```python
from build123d import *

# Parameters (mm, degrees)
SKETCH009_W          = 140
SKETCH009_H          = 120
PAD004_DEPTH         = 14
POCKET005_DEPTH      = 12
SKETCH011_R          = 1.75
POCKET006_DEPTH      = 0.001
POCKET006_DEPTH_BACK = 14.001
SKETCH012_R          = 4
POCKET007_DEPTH      = 12.001
SKETCH013_R          = 1.75
POCKET008_DEPTH      = 14.001


with BuildPart() as part:
    # Sketch009 → Pad004 (new body)
    with BuildSketch(Plane.XY):
        with Locations((-11.165, 15.85)):
            Rectangle(SKETCH009_W, SKETCH009_H)
    extrude(amount=PAD004_DEPTH)

    # Sketch010 → Pocket005 (cut)
    with BuildSketch(Plane.XY):
        with BuildLine():
            ThreePointArc((-79.165, 60.35), (-69.619058, 64.304058), (-65.665, 73.85))
            Line((43.335, 73.85), (-65.665, 73.85))
            ThreePointArc((43.335, 73.85), (47.289058, 64.304058), (56.835, 60.35))
            Line((56.835, -42.15), (56.835, 60.35))
            Line((-65.665, -42.15), (56.835, -42.15))
            ThreePointArc((-65.665, -42.15), (-69.619058, -32.604058), (-79.165, -28.65))
            Line((-79.165, 60.35), (-79.165, -28.65))
        make_face()
    extrude(amount=POCKET005_DEPTH, mode=Mode.SUBTRACT)

    # Sketch011 → Pocket006 (cut, two sides)
    with BuildSketch(Plane.XY) as pocket006_sk:
        with Locations((-74, 68)):
            Circle(SKETCH011_R)
        with Locations((52, 68)):
            Circle(SKETCH011_R)
        with Locations((-74, -37)):
            Circle(SKETCH011_R)
    extrude(amount=-POCKET006_DEPTH, mode=Mode.SUBTRACT)
    extrude(pocket006_sk.sketch, amount=POCKET006_DEPTH_BACK, mode=Mode.SUBTRACT)

    # Sketch012 (on DatumPlane) → Pocket007 (cut, through all)
    with BuildSketch(Plane.XY.offset(2)):
        with Locations((-74, 68)):
            Circle(SKETCH012_R)
        with Locations((52, 68)):
            Circle(SKETCH012_R)
        with Locations((-74, -37)):
            Circle(SKETCH012_R)
    extrude(amount=POCKET007_DEPTH, mode=Mode.SUBTRACT)

    # Sketch013 → Pocket008 (cut, through all)
    with BuildSketch(Plane.XY):
        with Locations((-36, 41)):
            Circle(SKETCH013_R)
        with Locations((-4, 41)):
            Circle(SKETCH013_R)
        with Locations((-36, 9)):
            Circle(SKETCH013_R)
        with Locations((-4, 9)):
            Circle(SKETCH013_R)
        with BuildLine():
            ThreePointArc((-40.582576, 39), (-32.464466, 37.464466), (-34, 45.582576))
            Line((-34, 45.582576), (-6, 45.582576))
            ThreePointArc((-6, 45.582576), (-7.535534, 37.464466), (0.582576, 39))
            Line((0.582576, 39), (0.582576, 11))
            ThreePointArc((0.582576, 11), (-7.535534, 12.535534), (-6, 4.417424))
            Line((-6, 4.417424), (-34, 4.417424))
            ThreePointArc((-34, 4.417424), (-32.464466, 12.535534), (-40.582576, 11))
            Line((-40.582576, 39), (-40.582576, 11))
        make_face()
    extrude(amount=POCKET008_DEPTH, mode=Mode.SUBTRACT)


with BuildPart() as part_1:
    # Body001 placement: moved
    add(part.part.moved(Location((0, 0, 32))))


solid = part_1.part
```
Geometry check sheet. Reference: the model listing, model coordinates, mm. A direction names the side the tool comes from. Round coordinates to 2 decimals unless told otherwise and drop trailing zeros. Write each loop counter-clockwise with the first axis right and the second up, starting at its lowest first coordinate (ties: lowest second). Pieces come first, ordered by that corner, then holes. Notation, with made-up numbers: (70.5, -4) - (120.5, -4) arc R17 ccw to (120.5, 3) - close; hole circle Ø10 at (82.25, 64). An arc over 180 degrees is marked (long way). Write each question's results on one line, items separated by ' | '.
(1) Sectioned sample at D-D, the plane x = -62. Enter the section's corners in (y, z).
Computed:
outline: (-44.15, 32) - (-42.15, 32) - (-42.15, 44) - (73.85, 44) - (73.85, 32) - (75.85, 32) - (75.85, 46) - (-44.15, 46) - close
(2) Sectioned sample at A-A, the plane x = -36. Enter the section's corners in (y, z), plus the area to 3 significant figures.
Computed:
outline: (-44.15, 32) - (-42.15, 32) - (-42.15, 44) - (7.25, 44) - (7.25, 46) - (-44.15, 46) - close; (10.75, 44) - (14, 44) - (14, 46) - (10.75, 46) - close; (36, 44) - (39.25, 44) - (39.25, 46) - (36, 46) - close; (42.75, 44) - (73.85, 44) - (73.85, 32) - (75.85, 32) - (75.85, 46) - (42.75, 46) - close | area: 230 mm^2
(3) Depth check by flat-ended pin: pin 1 Ø8 at (x, y) = (30, 12.5) entering from -Z; pin 2 Ø9 at (x, y) = (52, 68) entering from -Z; pin 3 Ø3 at (x, y) = (52, 68) entering from -Z; pin 4 Ø5.5 at (x, y) = (-74, 68) entering from +Z. Enter the tip coordinate at first touch or a pass-through.
Computed:
pin 1: stops at z = 44 | pin 2: stops at z = 32 | pin 3: passes through | pin 4: stops at z = 34
(4) Set-up check for faces 1 (the face through (51.133, 64.095, 39.916)), 2 (the face through (-72.331, -36.474, 32.986)), 3 (the face through (-10, 73.85, 38)): record each of +Z, -Z, +X, -X, +Y, -Y from which the full face is reachable in a straight line by a thin tool's end or side.
Computed:
face 1: +Z | face 2: +Z, -Z | face 3: -Z
(5) Sectioned sample at C-C, the plane y = 68. Enter the section's corners in (x, z) (3 decimals), plus the area to 3 significant figures.
Computed:
outline: (-81.165, 32) - (-75.75, 32) - (-75.75, 34) - (-78, 34) - (-78, 46) - (-81.165, 46) - close; (-72.25, 32) - (-66.998, 32) - (-66.998, 44) - (44.668, 44) - (44.668, 32) - (50.25, 32) - (50.25, 34) - (48, 34) - (48, 46) - (-70, 46) - (-70, 34) - (-72.25, 34) - close; (53.75, 32) - (58.835, 32) - (58.835, 46) - (56, 46) - (56, 34) - (53.75, 34) - close | area: 414 mm^2
(6) Thickness scan on probe 1 along Y at (x, z) = (-4, 44.65); probe 2 along X at (y, z) = (57, 38.25) (3 decimals); probe 3 along Y at (x, z) = (-23.5, 45.25). Record the ranges inside material, lowest first. Write a range as from..to.
Computed:
probe 1: y = -44.15..7.25, 10.75..14, 36..39.25, 42.75..75.85 | probe 2: x = -81.165..-79.165, 56.835..58.835 | probe 3: y = -44.15..4.42, 45.58..75.85
(7) Sectioned sample at B-B, the plane y = 41. Enter the section's corners in (x, z) (3 decimals), plus the area to 3 significant figures.
Computed:
outline: (-81.165, 32) - (-79.165, 32) - (-79.165, 44) - (-37.75, 44) - (-37.75, 46) - (-81.165, 46) - close; (-34.25, 44) - (-31, 44) - (-31, 46) - (-34.25, 46) - close; (-9, 44) - (-5.75, 44) - (-5.75, 46) - (-9, 46) - close; (-2.25, 44) - (56.835, 44) - (56.835, 32) - (58.835, 32) - (58.835, 46) - (-2.25, 46) - close | area: 270 mm^2
